Could you check a few things on this model? Use its own coordinates, in mm. Coordinates: 2 decimals unless noted, no trailing zeros. Write each loop counter-clockwise with the first axis right and the second up, starting at its lowest first coordinate (ties: lowest second). Pieces come first, ordered by that corner, then holes. Notation, with made-up numbers: (88.5, -35) - (103.5, -35) arc R26 ccw to (103.5, -18) - close; hole circle Ø4 at (-5.75, -38.75). An arc over 180 degrees is marked (long way). Write item = value, one per line. Start each with the question number.
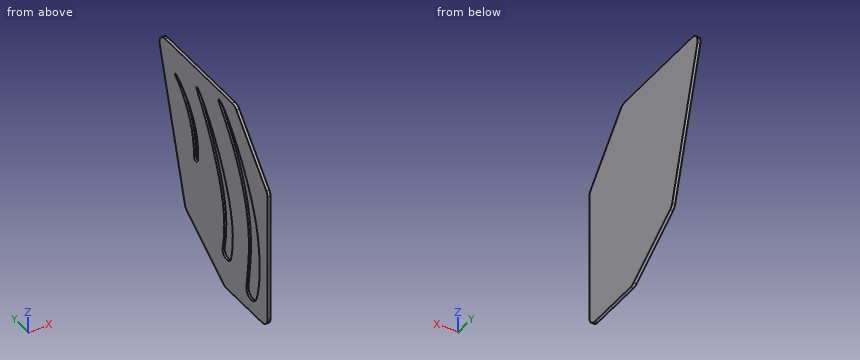
```python
from build123d import *

# Parameters (mm, degrees)
BOSS_EXTRUDE1_DEPTH = 10
CUT_EXTRUDE3_DEPTH  = 7


with BuildPart() as part:
    # Sketch1 → Boss-Extrude1 (new body)
    with BuildSketch(Plane(origin=(0, 0, 0), x_dir=(0, 0, -1), z_dir=(1, 0, 0))):
        with BuildLine():
            Line((0, -39.159060238), (0, -399.159060238))
            ThreePointArc((0, -399.159060238), (2.810766389, -411.83760809), (10.716371709, -422.140393531))
            Line((10.716371709, -422.140393531), (202.227482489, -582.837295953))
            ThreePointArc((202.227482489, -582.837295953), (211.25050648, -588.046741283), (221.51111078, -589.855962659))
            Line((221.51111078, -589.855962659), (671.51111078, -589.855962659))
            ThreePointArc((671.51111078, -589.855962659), (692.724314215, -581.069166095), (701.51111078, -559.855962659))
            Line((701.51111078, -559.855962659), (701.51111078, -369.855962659))
            ThreePointArc((701.51111078, -369.855962659), (700.081380744, -360.705024227), (695.928465834, -352.426310564))
            Line((695.928465834, -352.426310564), (556.491249073, -157.087470131))
            ThreePointArc((556.491249073, -157.087470131), (549.188422732, -149.877866821), (539.883012979, -145.551320648))
            Line((539.883012979, -145.551320648), (37.809118961, -10.19325866))
            ThreePointArc((37.809118961, -10.19325866), (11.755460664, -15.344426409), (0, -39.159060238))
        make_face()
    extrude(amount=BOSS_EXTRUDE1_DEPTH)

    # Sketch5 → Cut-Extrude3 (cut)
    with BuildSketch(Plane.ZY):
        with BuildLine():
            ThreePointArc((-331.179728441, -194.685467652), (-341.545058852, -204.318697463), (-332.693478174, -215.359019498))
            add(Edge.make_bspline(
                [(-332.693478174, -215.359019498), (-331.921739283, -215.472572374), (-226.918714052, -224.562098265), (-126.325036043, -154.802617957), (-92.163413905, -98.198220596)],
                knots=[0, 0, 0, 0, 0.354260741, 1, 1, 1, 1], degree=3))
            ThreePointArc((-92.163413905, -98.198220596), (-93.433821546, -92.827514339), (-98.829146805, -93.988930122))
            add(Edge.make_bspline(
                [(-98.829146805, -93.988930122), (-112.622758483, -114.88285895), (-192.730208888, -182.13783781), (-300.184384568, -194.688304583), (-331.179728441, -194.685467652)],
                knots=[0, 0, 0, 0, 0.660882752, 1, 1, 1, 1], degree=3))
        make_face()
        with BuildLine():
            ThreePointArc((-626.364411935, -475.947865394), (-654.270375926, -492.315038086), (-646.133694128, -523.626722446))
            add(Edge.make_bspline(
                [(-646.133694128, -523.626722446), (-620.265200397, -544.090123727), (-324.808789115, -589.015611509), (-14.475713482, -342.918185901), (-34.207392898, -327.560917886)],
                knots=[0, 0, 0, 0, 0.454280693, 1, 1, 1, 1], degree=3))
            ThreePointArc((-34.207392898, -327.560917886), (-38.301805286, -326.1553415), (-42.396217675, -327.560917886))
            add(Edge.make_bspline(
                [(-42.396217675, -327.560917886), (-179.998241324, -434.657283692), (-369.496171973, -510.067463814), (-572.427382245, -482.279425386), (-626.364411935, -475.947865394)],
                knots=[0, 0, 0, 0, 0.742688993, 1, 1, 1, 1], degree=3))
        make_face()
        with BuildLine():
            ThreePointArc((-567.085033992, -348.175125638), (-594.800287265, -365.58541059), (-577.755509271, -393.526935767))
            add(Edge.make_bspline(
                [(-577.755509271, -393.526935767), (-509.639726303, -410.500517765), (-300.322217315, -390.035120939), (-100.320017518, -254.957400328), (-66.698936736, -215.359019498)],
                knots=[0, 0, 0, 0, 0.345289595, 1, 1, 1, 1], degree=3))
            ThreePointArc((-66.698936736, -215.359019498), (-67.092959072, -208.260098077), (-74.202765192, -208.284508838))
            add(Edge.make_bspline(
                [(-74.202765192, -208.284508838), (-81.149231878, -214.924232147), (-316.076431581, -369.790908175), (-526.742508558, -357.109499901), (-567.085033992, -348.175125638)],
                knots=[0, 0, 0, 0, 0.768435057, 1, 1, 1, 1], degree=3))
        make_face()
    extrude(amount=-CUT_EXTRUDE3_DEPTH, mode=Mode.SUBTRACT)


solid = part.part
```
1) For P1, Ø1, axis at x = 1.5, z = -213.5, coming from the +Y side; P2, Ø6, axis at y = -404.5, z = -83, coming from the -X side; P3, Ø4, axis at y = -395, z = -448.5, coming from the -X side, each with a flat end and sliding along its axis, tell me the tip position at first contact or that it passes through.
2) Suppose I cut it at A-A on y = -53.5. Please give me the cut outline in (x, z), plus the area to 3 significant figures.
3) Suppose I cut it at B-B on x = 4.25. State how many separate pieces and enclosed holes the cut face has, plus the area to 3 significant figures.
4) If I drill on probe 1 along Y at (x, z) = (1.25, -328); probe 2 along Y at (x, z) = (2.5, -207.5); probe 3 along X at (y, z) = (-174.5, -182), over which ranges is the centre line in solid material (lowest first)? Write a range as [from, to].
Reply:
q1.P1 = -57.42
q1.P2 = 0
q1.P3 = 7
q2.outline = (0, -198.44) - (10, -198.44) - (10, 0) - (0, 0) - close
q2.area = 1,980 mm^2
q3.separate_pieces = 1
q3.enclosed_holes = 3
q3.area = 263,000 mm^2
q4.probe_1 = [-589.86, -518.42], [-473.14, -370.28], [-331.79, -215.71], [-194.67, -88.43]
q4.probe_2 = [-586.38, -465.83], [-430.34, -315.69], [-283.96, -196.51], [-171.47, -55.94]
q4.probe_3 = [7, 10]
